```python
from build123d import *

# Parameters (mm, degrees)
SKETCH1_R                      = 2.794
BOSS_EXTRUDE1_DEPTH            = 4.6355
SKETCH3_W                      = 5.2705
SKETCH3_H                      = 10.4775
BOSS_EXTRUDE3_DEPTH            = 7.366
SKETCH5_R                      = 1.651
CUT_EXTRUDE2_DEPTH             = 15.8115
CUT_EXTRUDE3_REACH             = 4.731
SKETCH6_W                      = 25.4
SKETCH6_H                      = 2.54
CUT_EXTRUDE3_DIRECTION_2_REACH = 14.002
FILLET1_R                      = 0.762


with BuildPart() as part:
    # Sketch1 → Boss-Extrude1 (new body, symmetric)
    with BuildSketch(Plane(origin=(0, 0, 0), x_dir=(1, 0, 0), z_dir=(0, 1, 0))):
        Polygon((-11.1125, 3.81), (-4.191, 3.81), (-4.191, 9.144), (14.2875, 9.144), (14.2875, -6.6675), (-11.1125, -6.6675), align=None)
        Circle(SKETCH1_R, mode=Mode.SUBTRACT)
    extrude(amount=BOSS_EXTRUDE1_DEPTH, both=True)

    # Sketch3 → Boss-Extrude3 (add, symmetric)
    with BuildSketch(Plane(origin=(0, 0, 0), x_dir=(1, 0, 0), z_dir=(0, 1, 0))):
        with Locations((-8.47725, -1.42875)):
            Rectangle(SKETCH3_W, SKETCH3_H)
    extrude(amount=BOSS_EXTRUDE3_DEPTH, both=True)

    # Sketch5 → Cut-Extrude2 (cut)
    with BuildSketch(Plane.XY.offset(6.6675)):
        with Locations((9.2075, 0)):
            Circle(SKETCH5_R)
    extrude(amount=-CUT_EXTRUDE2_DEPTH, mode=Mode.SUBTRACT)

    # Cut-Extrude3: up to this face of the body (flat: up to its plane)
    cut_extrude3_end = Plane(part.part.faces().sort_by_distance((-8.47725, 7.366, 1.42875))[0])
    # Sketch6 → Cut-Extrude3 (cut, up to the picked face)
    with BuildSketch(Plane(origin=(0, 4.6355, 0), x_dir=(1, 0, 0), z_dir=(0, 1, 0)), mode=Mode.PRIVATE) as cut_extrude3_sk1:
        with Locations((1.5875, -5.3975)):
            Rectangle(SKETCH6_W, SKETCH6_H)
    cut_extrude3_tool1 = split(extrude(cut_extrude3_sk1.sketch, amount=CUT_EXTRUDE3_REACH, mode=Mode.PRIVATE), bisect_by=cut_extrude3_end, keep=Keep.BOTH, mode=Mode.PRIVATE)
    add(cut_extrude3_tool1.solids().sort_by_distance((1.5875, 4.6355, 5.3975))[0], mode=Mode.SUBTRACT)

    # Cut-Extrude3 direction 2: up to this face of the body (flat: up to its plane)
    cut_extrude3_direction_2_end = Plane(part.part.faces().sort_by_distance((-8.47725, -7.366, 1.42875))[0])
    # Sketch6 → Cut-Extrude3 direction 2 (cut, up to the picked face)
    with BuildSketch(Plane(origin=(0, 4.6355, 0), x_dir=(1, 0, 0), z_dir=(0, 1, 0)), mode=Mode.PRIVATE) as cut_extrude3_direction_2_sk1:
        with Locations((1.5875, -5.3975)):
            Rectangle(SKETCH6_W, SKETCH6_H)
    cut_extrude3_direction_2_tool1 = split(extrude(cut_extrude3_direction_2_sk1.sketch, amount=-CUT_EXTRUDE3_DIRECTION_2_REACH, mode=Mode.PRIVATE), bisect_by=cut_extrude3_direction_2_end, keep=Keep.BOTH, mode=Mode.PRIVATE)
    add(cut_extrude3_direction_2_tool1.solids().sort_by_distance((1.5875, 4.6355, 5.3975))[0], mode=Mode.SUBTRACT)

    # Fillet1
    fillet1_edges = [part.edges().sort_by_distance(p)[0] for p in [
        (-11.1125, 0, -3.81),
        (-4.191, 0, -3.81),
        (-4.191, 0, -9.144),
        (14.2875, 0, -9.144),
        (5.04825, 4.6355, -9.144),
        (-4.191, 4.6355, -6.477),
        (-5.0165, 4.6355, -3.81),
        (-5.842, 6.00075, -3.81),
        (-5.842, -6.00075, -3.81),
        (-8.47725, -7.366, -3.81),
        (-11.1125, -7.366, 0.15875),
        (-8.47725, 7.366, -3.81),
        (-11.1125, 7.366, 0.15875),
        (-5.842, 7.366, 0.15875),
        (-5.842, -7.366, 0.15875),
        (14.2875, -4.6355, -2.50825),
        (14.2875, 4.6355, -2.50825),
        (-8.47725, -7.366, 4.1275),
        (-8.47725, 7.366, 4.1275),
        (-5.0165, -4.6355, -3.81),
        (-5.842, -6.00075, 4.1275),
        (14.2875, 0, 4.1275),
        (4.22275, -4.6355, 4.1275),
        (4.22275, 4.6355, 4.1275),
        (-5.842, 6.00075, 4.1275),
        (-11.1125, 0, 4.1275),
        (-4.191, -4.6355, -6.477),
        (5.04825, -4.6355, -9.144),
    ]]
    fillet(fillet1_edges, radius=FILLET1_R)


solid = part.part
```
Build history of the part. All positions in model axes, mm. A direction names the side the tool comes from. Give positions to 0.01 mm unless a question says otherwise; leave off trailing zeros. Order: outer loops, then holes, each group sorted by start corner. A loop starts at its lowest first (then second) coordinate and runs counter-clockwise, first axis right, second up. Notation, with made-up numbers: M 4,86.5 L 45,86.5 A34 ccw 45,123.5 Z; hole C 61.25,29 d5. An arc over 180 degrees is marked long. Return JSON: item names as keys, results as strings.
Q1. Wall check: probe 1 along Z at (x, y) = (0, -0.75); probe 2 along X at (y, z) = (1, -0.5); probe 3 along Y at (x, z) = (0.75, -6.5). Give the ranges that are in metal, low to high. Write a range as from..to.
Answer list:
{"probe 1": "z = -9.14..-2.79, 2.79..4.13", "probe 2": "x = -11.11..-2.75, 2.75..7.89, 10.52..14.29", "probe 3": "y = -4.64..4.64"}
Q2. Band-saw the part on D-D (z = -6.5). Give the cut face in (x, y).
Answer list:
{"outline": "M -4.19,-3.87 A0.76 ccw -3.43,-4.64 L 13.53,-4.64 A0.76 ccw 14.29,-3.87 L 14.29,3.87 A0.76 ccw 13.53,4.64 L -3.43,4.64 A0.76 ccw -4.19,3.87 Z; hole C 9.21,0 d3.3"}
Q3. Band-saw the part on B-B (z = 0). Give the cut face in (x, y).
Answer list:
{"outline": "M -11.11,-6.6 A0.76 ccw -10.35,-7.37 L -6.6,-7.37 A0.76 ccw -5.84,-6.6 L -5.84,-4.64 L -2.79,-4.64 L -2.79,4.64 L -5.84,4.64 L -5.84,6.6 A0.76 ccw -6.6,7.37 L -10.35,7.37 A0.76 ccw -11.11,6.6 Z; M 2.79,-4.64 L 13.53,-4.64 A0.76 ccw 14.29,-3.87 L 14.29,3.87 A0.76 ccw 13.53,4.64 L 2.79,4.64 Z; hole C 9.21,0 d3.3"}
Q4. Band-saw the part on A-A (y = 0). Give the cut face in (x, z).
Answer list:
{"outline": "M -11.11,-3.05 A0.76 ccw -10.35,-3.81 L -4.95,-3.81 A0.76 cw -4.19,-4.57 L -4.19,-8.38 A0.76 ccw -3.43,-9.14 L 7.56,-9.14 L 7.56,4.13 L -10.35,4.13 A0.76 ccw -11.11,3.37 Z; M 10.86,-9.14 L 13.53,-9.14 A0.76 ccw 14.29,-8.38 L 14.29,3.37 A0.76 ccw 13.53,4.13 L 10.86,4.13 Z; hole C 0,0 d5.59"}
Q5. Band-saw the part on C-C (x = 0). Give the cut face in (y, z).
Answer list:
{"outline": "M -4.64,-8.38 A0.76 ccw -3.87,-9.14 L 3.87,-9.14 A0.76 ccw 4.64,-8.38 L 4.64,-2.79 L -4.64,-2.79 Z; M -4.64,2.79 L 4.64,2.79 L 4.64,3.37 A0.76 ccw 3.87,4.13 L -3.87,4.13 A0.76 ccw -4.64,3.37 Z"}
Q6. 3-axis set-ups, long thin cutter, end or side, ignore diameter. For faces 1 (the face through (6, -4.636, -3)), 2 (the face through (5, 0, -9.144)), 3 (the face through (-8, 0, -3.81)), 4 (the face through (-5.842, 6, 0)): which of +Z, -Z, +X, -X, +Y, -Y reach the whole face in a straight line?
Answer list:
{"face 1": "+Z, -Z, +X, -Y", "face 2": "-Z, +X, -X, +Y, -Y", "face 3": "-Z, -X, +Y, -Y", "face 4": "+Z, -Z, +X, +Y"}
Q7. Two-plate mould, pull along Z, no slides. Class faces 5 (the face through (-2.217, -0.065, 1.7)), 6 (the face through (7.897, -1.005, -2.415)), 7 (the face through (-1, 0, 4.127)): pulls with the +Z half, pulls with the -Z half, needs draft (parallel to the pull), parting line crosses it, or undercut.
Answer list:
{"face 5": "undercut", "face 6": "needs draft", "face 7": "pulls with the +Z half"}
Q8. Flat gauge pins, fed straight in: pin 1 (3 mm diameter, centred on x = -7.5, y = -2, fed in from -Z); pin 2 (6 mm diameter, centred on x = 1, z = -1.5, fed in from -Y); pin 3 (1.6 mm diameter, centred on y = 6, z = -1, fed in from +X); pin 4 (1 mm diameter, centred on x = -8, z = -5.5, fed in from +Y). Where does each tip first touch, or does it go through?
Answer list:
{"pin 1": "stops at z = -3.81", "pin 2": "stops at y = -4.64", "pin 3": "stops at x = -5.84", "pin 4": "passes through"}
